Read the model definition and answer for the solid it produces. Units are mm, in the model's axes. A direction names the side the tool comes from. Coordinates: 2 decimals unless noted, no trailing zeros. Order: outer loops, then holes, each group sorted by start corner. A loop starts at its lowest first (then second) coordinate and runs counter-clockwise, first axis right, second up.
from build123d import *

# Parameters (mm, degrees)
SKETCH1_R           = 0.625
SKETCH1_R_2         = 1.265
BOSS_EXTRUDE2_DEPTH = 1.95
BOSS_EXTRUDE3_START = -1.4
BOSS_EXTRUDE3_DEPTH = 1.4
BOSS_EXTRUDE4_DEPTH = 3.7
CUT_EXTRUDE1_START  = -1
SKETCH4_R           = 2.315
SKETCH4_R_2         = 1.265
CUT_EXTRUDE1_DEPTH  = 1


with BuildPart() as part:
    # Sketch1 → Boss-Extrude2 (new body)
    with BuildSketch(Plane(origin=(0, 0, 0), x_dir=(1, 0, 0), z_dir=(0, 1, 0))):
        with BuildLine():
            Line((-2.4, 15.5), (-3.557102073, 0.554098225))
            ThreePointArc((-3.557102073, 0.554098225), (0, -3.6), (3.557102073, 0.554098225))
            Line((3.557102073, 0.554098225), (2.4, 15.5))
            ThreePointArc((2.4, 15.5), (0, 17.9), (-2.4, 15.5))
        make_face()
        with Locations(Location((0, 5.775, 0), (0, 0, 270))):
            Circle(SKETCH1_R, mode=Mode.SUBTRACT)
        with Locations(Location((0, 8.325, 0), (0, 0, 270))):
            Circle(SKETCH1_R, mode=Mode.SUBTRACT)
        with Locations(Location((0, 10.875, 0), (0, 0, 270))):
            Circle(SKETCH1_R, mode=Mode.SUBTRACT)
        with Locations(Location((0, 13.425, 0), (0, 0, 270))):
            Circle(SKETCH1_R, mode=Mode.SUBTRACT)
        with Locations(Location((0, 15.975, 0), (0, 0, 270))):
            Circle(SKETCH1_R, mode=Mode.SUBTRACT)
        with Locations(Location((0, 0, 0), (0, 0, 270))):
            Circle(SKETCH1_R_2, mode=Mode.SUBTRACT)
    extrude(amount=BOSS_EXTRUDE2_DEPTH)

    # Sketch1_4 → Boss-Extrude3 (add)
    with BuildSketch(Plane(origin=(0, 0, 0), x_dir=(1, 0, 0), z_dir=(0, 1, 0)).offset(BOSS_EXTRUDE3_START)):
        with BuildLine():
            Line((0, -2.315), (0, -3.6))
            ThreePointArc((0, -3.6), (2.545584412, -2.545584412), (3.6, 0))
            Line((3.6, 0), (3.557102073, 0.554098225))
            ThreePointArc((3.557102073, 0.554098225), (2.341500202, 2.734479257), (0, 3.6))
            Line((0, 3.6), (0, 2.315))
            ThreePointArc((0, 2.315), (1.636952198, 1.636952198), (2.315, 0))
            ThreePointArc((2.315, 0), (1.636952198, -1.636952198), (0, -2.315))
        make_face()
        with BuildLine():
            ThreePointArc((-3.6, 0), (-2.545584412, -2.545584412), (0, -3.6))
            Line((0, -3.6), (0, -2.315))
            ThreePointArc((0, -2.315), (-2.315, 0), (0, 2.315))
            Line((0, 2.315), (0, 3.6))
            ThreePointArc((0, 3.6), (-2.341500202, 2.734479257), (-3.557102073, 0.554098225))
            Line((-3.557102073, 0.554098225), (-3.6, 0))
        make_face()
    extrude(amount=BOSS_EXTRUDE3_DEPTH)

    # Sketch1_5 → Boss-Extrude4 (add)
    with BuildSketch(Plane(origin=(0, 0, 0), x_dir=(1, 0, 0), z_dir=(0, 1, 0))):
        with BuildLine():
            Line((0, -2.315), (0, -3.6))
            ThreePointArc((0, -3.6), (2.545584412, -2.545584412), (3.6, 0))
            Line((3.6, 0), (3.557102073, 0.554098225))
            ThreePointArc((3.557102073, 0.554098225), (2.341500202, 2.734479257), (0, 3.6))
            Line((0, 3.6), (0, 2.315))
            ThreePointArc((0, 2.315), (1.636952198, 1.636952198), (2.315, 0))
            ThreePointArc((2.315, 0), (1.636952198, -1.636952198), (0, -2.315))
        make_face()
        with BuildLine():
            ThreePointArc((-3.6, 0), (-2.545584412, -2.545584412), (0, -3.6))
            Line((0, -3.6), (0, -2.315))
            ThreePointArc((0, -2.315), (-2.315, 0), (0, 2.315))
            Line((0, 2.315), (0, 3.6))
            ThreePointArc((0, 3.6), (-2.341500202, 2.734479257), (-3.557102073, 0.554098225))
            Line((-3.557102073, 0.554098225), (-3.6, 0))
        make_face()
    extrude(amount=BOSS_EXTRUDE4_DEPTH)

    # Sketch4 → Cut-Extrude1 (cut)
    with BuildSketch(Plane(origin=(0, 1.95, 0), x_dir=(1, 0, 0), z_dir=(0, 1, 0)).offset(CUT_EXTRUDE1_START)):
        with Locations(Location((0, 0, 0), (0, 0, 270))):
            Circle(SKETCH4_R)
        with Locations(Location((0, 0, 0), (0, 0, 270))):
            Circle(SKETCH4_R_2, mode=Mode.SUBTRACT)
    extrude(amount=CUT_EXTRUDE1_DEPTH, mode=Mode.SUBTRACT)


solid = part.part
Q1. Straight lines are drawn through the part: L1, parallel to X at y = 1.35, z = 0 (3 decimals); L2, parallel to Y at x = 0, z = -14.75; L3, parallel to X at y = 3.1, z = 1.5. For each, find the intervals that lie inside material, in ascending order.
Q2. The part is cut by section C-C, the plane y = 0.5. Determine the outline of the cut face in (x, z) (3 decimals).
Q3. Each of these flat-tipped pins is pushed along its axis until it touches: P1, Ø1, axis at x = 2, y = -0.5, coming from the +Z side; P2, Ø0.8, axis at x = 0, z = -15.975, coming from the -Y side; P3, Ø3.5, axis at x = -0.5, z = 1, coming from the -Y side; P4, Ø2, axis at y = 3, z = -2.5, coming from the +X side. Where does it stop, or does it pass through?
Q4. The part is cut by section D-D, the plane x = 1.5. Determine the outline of the cut face in (y, z), then the cut area to 3 significant figures.
Q5. The part is cut by section A-A, the plane y = 2.15. Determine the outline of the cut face in (x, z) (3 decimals).
Q6. The part is cut by section B-B, the plane z = -16. Determine the outline of the cut face in (x, y).
Q7. Which of the six approach directions +Z, -Z, +X, -X, +Y, -Y give full straight-line access (tool end or side, diameter ignored) to faces 4 (the cylindrical face through (-0.24, 0.96, -5.2)), 5 (the flat face through (0, 0, 2)), 6 (the flat face through (-2, 0.95, 0))?
Q8. Determine the mould class of faces 1 (the cylindrical face through (0.4, 0.5, 1.2)), 2 (the flat face through (2.35, -1.4, 0.75)), 3 (the flat face through (2.987, 0.961, -7.922)) for opening direction X: +X half, -X half, draft (parallel to the pull), parting line (faces both ways), or undercut.
Computed values:
1. L1: x = -3.6 to -2.315, 2.315 to 3.6
1. L2: y = 0 to 1.95
1. L3: x = -3.27 to -1.76, 1.76 to 3.27
2. outline: (-3.557, -0.554) - (-2.4, -15.5) arc R2.4 ccw to (2.4, -15.5) - (3.557, -0.554) arc R3.6 ccw (long way) to start; hole circle Ø2.53 at (0, 0); hole circle Ø1.25 at (0, -15.975); hole circle Ø1.25 at (0, -13.425); hole circle Ø1.25 at (0, -10.875); hole circle Ø1.25 at (0, -8.325); hole circle Ø1.25 at (0, -5.775)
3. P1: stops at z = 3.27
3. P2: passes through
3. P3: stops at y = -1.4
3. P4: stops at x = 3.27
4. outline: (-1.4, -3.27) - (0, -3.27) - (0, -17.37) - (1.95, -17.37) - (1.95, -3.27) - (3.7, -3.27) - (3.7, -1.76) - (0.95, -1.76) - (0.95, 1.76) - (3.7, 1.76) - (3.7, 3.27) - (-1.4, 3.27) - (-1.4, 1.76) - (0, 1.76) - (0, -1.76) - (-1.4, -1.76) - close
4. area: 46.2 mm2
5. outline: (-3.6, 0) - (-3.557, -0.554) arc R3.6 ccw to (3.557, -0.554) - (3.6, 0) arc R3.6 ccw to start; hole circle Ø4.63 at (0, 0)
6. outline: (-2.35, 0) - (-0.62, 0) - (-0.62, 1.95) - (-2.35, 1.95) - close; (0.62, 0) - (2.35, 0) - (2.35, 1.95) - (0.62, 1.95) - close
7. face 4: +Y, -Y
7. face 5: -Y
7. face 6: +Y
8. face 1: undercut
8. face 2: draft
8. face 3: +X half
